from build123d import *

# Parameters (mm, degrees)
SKETCH1_R           = 1.65
SKETCH1_R_2         = 12.7
BOSS_EXTRUDE1_DEPTH = 6.35


with BuildPart() as part:
    # Sketch1 → Boss-Extrude1 (new body)
    with BuildSketch(Plane.XZ.offset(-50.8)):
        Polygon((-350.52, 222.25), (-350.52, 215.9), (-359.9825, 215.9), (-359.9825, 210.9), (-358.7825, 210.9), (-358.7825, 208.4), (-359.9825, 208.4), (-359.9825, 205.9), (-363.2825, 205.9), (-363.2825, 208.4), (-364.4825, 208.4), (-364.4825, 210.9), (-363.2825, 210.9), (-363.2825, 215.9), (-375.92, 215.9), (-375.92, 177.8), (-382.27, 177.8), (-382.27, 152.4), (-375.92, 152.4), (-375.92, 69.85), (-382.27, 69.85), (-382.27, 44.45), (-375.92, 44.45), (-375.92, -38.1), (-382.27, -38.1), (-382.27, -63.5), (-375.92, -63.5), (-375.92, -146.05), (-382.27, -146.05), (-382.27, -177.8), (-375.92, -177.8), (-375.92, -215.9), (-363.2825, -215.9), (-363.2825, -210.9), (-364.4825, -210.9), (-364.4825, -208.4), (-363.2825, -208.4), (-363.2825, -205.9), (-359.9825, -205.9), (-359.9825, -208.4), (-358.7825, -208.4), (-358.7825, -210.9), (-359.9825, -210.9), (-359.9825, -215.9), (-350.52, -215.9), (-350.52, -222.25), (-325.12, -222.25), (-325.12, -215.9), (-315.6575, -215.9), (-315.6575, -210.9), (-316.8575, -210.9), (-316.8575, -208.4), (-315.6575, -208.4), (-315.6575, -205.9), (-312.3575, -205.9), (-312.3575, -208.4), (-311.1575, -208.4), (-311.1575, -210.9), (-312.3575, -210.9), (-312.3575, -215.9), (-299.72, -215.9), (-299.72, 215.9), (-312.3575, 215.9), (-312.3575, 210.9), (-311.1575, 210.9), (-311.1575, 208.4), (-312.3575, 208.4), (-312.3575, 205.9), (-315.6575, 205.9), (-315.6575, 208.4), (-316.8575, 208.4), (-316.8575, 210.9), (-315.6575, 210.9), (-315.6575, 215.9), (-325.12, 215.9), (-325.12, 222.25), align=None)
        with Locations((-379.095, 165.1)):
            Circle(SKETCH1_R, mode=Mode.SUBTRACT)
        with Locations((-379.095, 57.15)):
            Circle(SKETCH1_R, mode=Mode.SUBTRACT)
        with Locations((-379.095, -161.925)):
            Circle(SKETCH1_R, mode=Mode.SUBTRACT)
        with Locations((-379.095, -50.8)):
            Circle(SKETCH1_R, mode=Mode.SUBTRACT)
        with Locations((-325.259000014, -13.688281448)):
            Circle(SKETCH1_R, mode=Mode.SUBTRACT)
        with Locations((-356.259000014, -13.688281448)):
            Circle(SKETCH1_R, mode=Mode.SUBTRACT)
        with Locations((-325.259000014, -44.688281448)):
            Circle(SKETCH1_R, mode=Mode.SUBTRACT)
        with Locations((-356.259000014, -44.688281448)):
            Circle(SKETCH1_R, mode=Mode.SUBTRACT)
        with Locations((-340.759000014, -29.188281448)):
            Circle(SKETCH1_R_2, mode=Mode.SUBTRACT)
    extrude(amount=-BOSS_EXTRUDE1_DEPTH)


solid = part.part
Verification items for the finished model (mm, model axes). Coordinates: 2 decimals unless noted, no trailing zeros. Write each loop counter-clockwise with the first axis right and the second up, starting at its lowest first coordinate (ties: lowest second). Pieces come first, ordered by that corner, then holes. Notation, with made-up numbers: (-28.75, 73.25) -> (-24.75, 73.25) arc R30 cw to (-24.75, 107.25) -> close; hole circle Ø1 at (-7, 87.25). An arc over 180 degrees is marked (long way). One line per item, written item: value. Start each with the question number.
Q1. Go/stop test with flat-tipped pins: P1, Ø1.2, axis at y = 54, z = -210, coming from the -X side; P2, Ø2, axis at x = -314.5, y = 53, coming from the +Z side; P3, Ø0.6, axis at x = -359.5, y = 52.5, coming from the +Z side; P4, Ø15, axis at x = -340.76, z = -29.19, coming from the -Y side (3 decimals). Record where each tip stops, or that it passes through.
Q2. Cross-section at C-C on y = 55.5. State how many separate pieces and enclosed holes the cut face has, and give its area (3 significant figures).
Q3. Cross-section at A-A on x = -343. Enter the section's corners in (y, z).
Q4. Cross-section at B-B on z = -139. Enter the section's corners in (x, y), and give its area (3 significant figures).
Q5. Mould release check, pull along X, two halves, no side actions. Record for faces 1 (the flat face through (-342, 57.15, 3)), 2 (the cylindrical face through (-350.837, 53.931, -36.916)): pulls with the +X half, pulls with the -X half, needs draft (parallel to the pull), parting line crosses it, or undercut.
Q6. Thickness scan on L1, parallel to Z at x = -363.5, y = 56; L2, parallel to Z at x = -376.5, y = 55.5; L3, parallel to Z at x = -341.5, y = 54.5. Record the ranges inside material, lowest first. Write a range as from..to.
Checked values:
1. P1: stops at x = -375.92
1. P2: stops at z = 205.9
1. P3: stops at z = 215.9
1. P4: passes through
2. separate pieces: 1
2. enclosed holes: 9
2. area: 33,200 mm²
3. outline: (50.8, -222.25) -> (57.15, -222.25) -> (57.15, -41.69) -> (50.8, -41.69) -> close; (50.8, -16.69) -> (57.15, -16.69) -> (57.15, 222.25) -> (50.8, 222.25) -> close
4. outline: (-375.92, 50.8) -> (-299.72, 50.8) -> (-299.72, 57.15) -> (-375.92, 57.15) -> close
4. area: 484 mm²
5. face 1: needs draft
5. face 2: undercut
6. L1: z = -215.9..-210.9, -208.4..208.4, 210.9..215.9
6. L2: z = -177.8..-146.05, -63.5..-38.1, 44.45..69.85, 152.4..177.8
6. L3: z = -222.25..-41.87, -16.51..222.25
